The model under review builds one solid part; all positions refer to its coordinate system, in mm. A direction names the side the tool comes from. Coordinates: 2 decimals unless noted, no trailing zeros. Write each loop counter-clockwise with the first axis right and the second up, starting at its lowest first coordinate (ties: lowest second). Pieces come first, ordered by that corner, then holes. Notation, with made-up numbers: (64.25, 86) - (99.25, 86) arc R21 ccw to (99.25, 93) - close; hole circle Ø1 at (2, 66). An arc over 180 degrees is marked (long way). Return JSON: item names as keys, results as strings. Group by question number.
(1) For pin 1 Ø3 at (x, y) = (0, 0.5) entering from -Z; pin 2 Ø3 at (x, y) = (0, 0) entering from +Z; pin 3 Ø1 at (y, z) = (-1.5, 6.5) entering from -X; pin 4 Ø4 at (x, z) = (4, 12) entering from -Y, all flat-tipped, find the tip position at first contact; note any pin that passes through.
(2) We need section A-A on z = 12. State the section outline as (x, y) points.
(3) Draft analysis for pull direction X (two halves, no side actions). For faces 5 (the face through (1.793, 1.743, 11.367)), 6 (the face through (0, -1, 11)), 7 (the face through (3, 0.1, 0.5)), 8 (the face through (-2.868, 2.789, 0.493)), state which applies: released by +X, released by -X, zero draft, split by the parting line, or undercut.
(4) Tool access review of faces 1 (the face through (-1.743, 1.793, 11.367)), 2 (the face through (1, 1, 1)), 3 (the face through (-1.793, -1.743, 11.367)), 4 (the face through (1.743, -1.793, 11.367)): name each direction out of +Z, -Z, +X, -X, +Y, -Y from which nothing blocks a thin tool from reaching the whole face with its end or side.
(5) To check wall thickness, follow L1, parallel to X at y = -0.25, z = 20.25; L2, parallel to Y at x = -0.5, z = 18.75; L3, parallel to X at y = 0.75, z = 10. State the ranges of each line that lie inside material, in increasing order. Write a range as from..to.
```python
from build123d import *

# Parameters (mm, degrees)
BASE_DEPTH          = 1
BOSS_EXTRUDE2_DEPTH = 20
SKETCH3_R           = 1
CUT_EXTRUDE1_DEPTH  = 23.472205054
FILLET1_R           = 1
SKETCH4_R           = 3
CUT_EXTRUDE2_DEPTH  = 1


with BuildPart() as part:
    # Sketch1 → Base (new body)
    with BuildSketch(Plane.XY):
        Polygon((-5.656854249, 0), (0, 5.656854249), (5.656854249, 0), (0, -5.656854249), align=None)
    extrude(amount=BASE_DEPTH)

    # Sketch2 → Boss-Extrude2 (add)
    with BuildSketch(Plane.XY.offset(1)):
        Polygon((0, -3.535533906), (3.535533906, 0), (0, 3.535533906), (-3.535533906, 0), align=None)
    extrude(amount=BOSS_EXTRUDE2_DEPTH)

    # Sketch3 → Cut-Extrude1 (cut, through all)
    with BuildSketch(Plane.XY.offset(21)):
        Circle(SKETCH3_R)
    extrude(amount=-CUT_EXTRUDE1_DEPTH, mode=Mode.SUBTRACT)

    # Fillet1
    fillet1_edges = [part.edges().sort_by_distance(p)[0] for p in [
        (-1.767766953, -1.767766953, 1),
        (1.767766953, -1.767766953, 1),
        (1.767766953, 1.767766953, 1),
        (-1.767766953, 1.767766953, 1),
    ]]
    fillet(fillet1_edges, radius=FILLET1_R)

    # Sketch4 → Cut-Extrude2 (cut)
    with BuildSketch(Plane(origin=(0, 0, 0), x_dir=(-1, 0, 0), z_dir=(0, 0, -1))):
        Circle(SKETCH4_R)
    extrude(amount=-CUT_EXTRUDE2_DEPTH, mode=Mode.SUBTRACT)


solid = part.part
```
Ans:
{
 "1": {"pin 1": "z = 1", "pin 2": "z = 21", "pin 3": "x = -2.54", "pin 4": "y = -1.54"},
 "2": {"outline": "(-3.54, 0) - (0, -3.54) - (3.54, 0) - (0, 3.54) - close; hole circle Ø2 at (0, 0)"},
 "3": {"face 5": "released by +X", "face 6": "undercut", "face 7": "undercut", "face 8": "released by -X"},
 "4": {"face 1": "+Z, -X, +Y", "face 2": "-Z", "face 3": "+Z, -X, -Y", "face 4": "+Z, +X, -Y"},
 "5": {"L1": "-3.29..-0.97, 0.97..3.29", "L2": "-3.04..-0.87, 0.87..3.04", "L3": "-2.79..-0.66, 0.66..2.79"}
}
